Could you check a few things on this model? Use its own coordinates, in mm. Face numbers are marked on the shaded views. Coordinates: 2 decimals unless noted, no trailing zeros. Order: outer loops, then holes, each group sorted by start corner. A loop starts at its lowest first (then second) coordinate and runs counter-clockwise, first axis right, second up. Notation, with made-up numbers: (8, 34) - (62, 34) arc R28 ccw to (62, 63) - close; hole circle Ø11 at (-37.5, 0.5). An arc over 180 degrees is marked (long way). One line per item, written item: value. Start each with the question number.
Autodesk Inventor part; units mm, degrees
ref_plane "Work Plane1" through (20, 0, 0) normal (0, 0.5, 0.866) x (1, 0, 0)
ref_plane "YZ Plane" through (0, 0, 0) normal (1, 0, 0) x (0, 1, 0)
ref_plane "XZ Plane" through (0, 0, 0) normal (0, 1, 0) x (-1, 0, 0)
sketch "Sketch1" plane through (0, 0, 0) normal (0, 0, 1) x (1, 0, 0)
  line L0 (0, 0) -> (33.6667, 0)
  line L1 (40, 2.3094) -> (40, 4)
  line L2 (40, 4) -> (0, 4)
  line L3 (40, 2.3094) -> (35, 2.3094)
  line L4 (35, 2.3094) -> (33.6667, 0)
  line L5 (0, -0.8) -> (0, 4.8)
  line L6 (0, 4) -> (0, 0)
  dimension "d0" = 5
  dimension "d1" = 60
  dimension "d2" = 8
  dimension "d3" = 4.6188
  dimension "d5" = 40
revolve "Body" add sketch "Sketch1" angle 360 about axis through (0, 0, 0) along (1, 0, 0)
chamfer "Chamfer1" distance 0.7668 angle 45 1 edges at (40, -4, 0) measured on face at (40, 3.3754, -0.5033)
sketch "Sketch2" plane through (40, 0, 0) normal (1, 0, 0) x (0, 0, -1)
  circle A0 centre (0, 0) radius 2.3094
  line L0 (-1.1547, 2) -> (1.1547, 2)
  line L1 (1.1547, 2) -> (2.3094, 0)
  line L2 (2.3094, 0) -> (1.1547, -2)
  line L3 (1.1547, -2) -> (-1.1547, -2)
  line L4 (-1.1547, -2) -> (-2.3094, 0)
  line L5 (-2.3094, 0) -> (-1.1547, 2)
extrude "Slot" add sketch "Sketch2" against normal up to next contours L1 A0 | A0 L2 | L0 A0 | A0 L3 | L5 A0 | A0 L4
thread "Thread"
chamfer "Chamfer2" distance 0.7668 angle 45 1 edges at (0, -4, 0) measured on face at (13.0777, 3.9482, -0.6416)
ref_plane "Work Plane1" through (20, 0, 0) normal (0, 0.5, 0.866) x (1, 0, 0)
equation "\"d7\" = -0.5 * GD1 + 0.5 * NND"
equation "\"d8\" = FAWI"
equation "\"d29\" = -0.5 * GD1 + 0.5 * NND"
equation "\"d11\" = NLG"
equation "\"d13\" = -0.5 * GD1 + 0.5 * NND"
equation "\"d14\" = FAWI"
equation "\"d30\" = -0.5 * GD1 + 0.5 * NND"
equation "\"d0\" = INTI"
equation "\"d2\" = NND"
equation "\"d3\" = 1.1547 * SW"
equation "\"d5\" = NLG"
equation "\"NND\" = 8"
equation "\"NLG\" = 40"
equation "\"INTI\" = 5"
equation "\"FAWI\" = 45deg"
equation "\"SW\" = 4"
equation "\"GD1\" = THREADDIA - 1.2269 * PTC"
equation "\"FAWI1\" = 45deg"
equation "\"GUL\" = 0.61345 * PTC"
equation "\"SPD\" = 5.5"
equation "\"SEWI\" = 90deg"
equation "\"TOA\" = 30deg"
equation "\"THREADDIA\" = 8"
equation "\"PTC\" = 1.25"
equation "\"GAL\" = 0.61345 * PTC"
equation "\"E0\" = 1.155 * SW"
properties part number "ISO 4026 - M8 x 40" material "Stainless Steel, 440C"
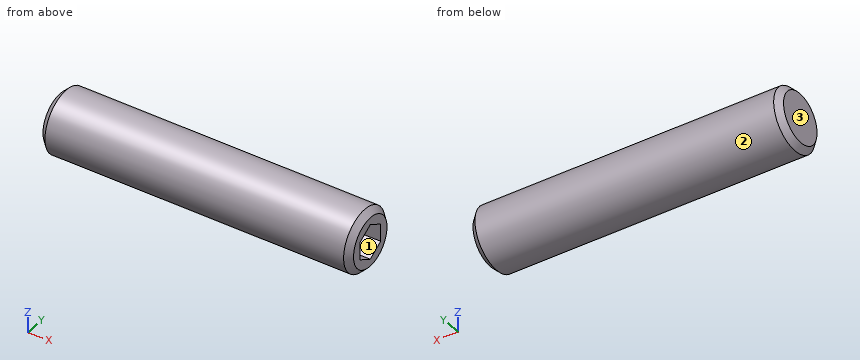
Q1. I'm going to push flat-ended pins straight in: pin 1 (4 mm diameter, centred on x = 11, y = -2, fed in from -Z); pin 2 (3 mm diameter, centred on x = 23.5, y = 2.5, fed in from +Z); pin 3 (3 mm diameter, centred on x = 23.5, y = 3, fed in from +Z); pin 4 (0.7 mm diameter, centred on x = 36.5, z = -0.5, fed in from +Y). Where does each tip first touch, or does it pass through?
Q2. If I drill on L1, parallel to Y at x = 36.5, z = -1.25; L2, parallel to Y at x = 12, z = -1.5; L3, parallel to Y at x = 25.5, z = -2.5, over which ranges is the centre line in solid material (lowest first)?
Q3. We'd pull the mould along Y, two halves only. Please class the marked faces 1, 2 and 3: +Y half, -Y half, draft (parallel to the pull), parting line (faces both ways), or undercut.
Q4. I want a section at A-A on x = 21.5. Please give me the cut outline in (y, z).
Values follow:
1. pin 1: stops at z = -4
1. pin 2: stops at z = 3.87
1. pin 3: stops at z = 3.71
1. pin 4: stops at y = 4
2. L1: y = -3.8 to -1.83, 1.83 to 3.8
2. L2: y = -3.71 to 3.71
2. L3: y = -3.12 to 3.12
3. face 1: undercut
3. face 2: parting line
3. face 3: draft
4. outline: circle Ø8 at (0, 0)
